Here's how the part is built. I have some questions about the finished solid (model axes, mm). A direction names the side the tool comes from. Coordinates: 2 decimals unless noted, no trailing zeros. Loops run counter-clockwise (first coordinate to the right, second up) from the corner with the lowest first, then second, coordinate; pieces in that order, holes last.
```python
from build123d import *

# Parameters (mm, degrees)
F0_R          = 15
F0_R_2        = 4
F1_DEPTH      = 2
F2_R          = 10.75
F2_R_2        = 4
F3_DEPTH      = 3
F4_R          = 1.5
F5_DEPTH      = 25
F5_DEPTH_BACK = 25
F6_R          = 1
F7_DEPTH      = 25


with BuildPart() as f1:
    # F0 (on Top) → F1 (new body)
    with BuildSketch(Plane.XY):
        Circle(F0_R)
        Circle(F0_R_2, mode=Mode.SUBTRACT)
    extrude(amount=F1_DEPTH)

    # F2 (on face) → F3 (join)
    with BuildSketch(Plane.XY.offset(2)):
        Circle(F2_R)
        Circle(F2_R_2, mode=Mode.SUBTRACT)
    extrude(amount=F3_DEPTH)

    # F4 (on Right) → F5 (cut, two sides)
    with BuildSketch(Plane.YZ) as f5_sk:
        with Locations((0, 2.5)):
            Circle(F4_R)
    extrude(amount=-F5_DEPTH, mode=Mode.SUBTRACT)
    extrude(f5_sk.sketch, amount=F5_DEPTH_BACK, mode=Mode.SUBTRACT)

    # F6 (on face) → F7 (cut)
    with BuildSketch(Plane.XY.offset(5)):
        with Locations((8.0107347155, -4.6250004669)):
            Circle(F6_R)
        with Locations((0, 9.25)):
            Circle(F6_R)
        with Locations((-8.0107355241, -4.6249990662)):
            Circle(F6_R)
    extrude(amount=-F7_DEPTH, mode=Mode.SUBTRACT)


solid = f1.part
```
1. I need wall thicknesses on line 1 along Y through (x, z) = (0, 2.5); line 2 along Y through (x, z) = (0, 1.6); line 3 along X through (y, z) = (-5.5, 1.2). Which ranges of each line are inside material? Lowest first, please.
2. I want a section at C-C (y = 0). Please give me the cut outline in (x, z), then the cut area to 3 significant figures.
3. We'd pull the mould along Z, two halves only. Please class faces 1 (the flat face through (3, -3, 0)), 2 (the cylindrical face through (8.02, 0.69, 1.17)), 3 (the flat face through (0, -5, 5)): +Z half, -Z half, draft (parallel to the pull), parting line (faces both ways), or undercut.
4. I want a section at D-D (y = 9.25). Please give me the cut outline in (x, z), then the cut area to 3 significant figures.
5. On a 3-axis mill with a long thin cutter (end or side, diameter ignored), from which of +Z, -Z, +X, -X, +Y, -Y can I reach the whole of each face in a straight line? I mean faces 4 (the cylindrical face through (7.01, -4.58, 2.54)), 5 (the flat face through (0, 11, 2)), 6 (the cylindrical face through (10.254, 3.229, 3.479)), 7 (the flat face through (0, -11, 2)). Say none if no direction works.
6. I want a section at B-B (z = 1.65). Please give me the cut outline in (x, y) (3 decimals).
7. I want a section at A-A (x = 0). Please give me the cut outline in (y, z), then the cut area to 3 significant figures.
Response values:
1. line 1: y = -10.75 to -4, 4 to 8.25, 10.25 to 10.75
1. line 2: y = -15 to -4, 4 to 8.25, 10.25 to 15
1. line 3: x = -13.96 to -8.49, -7.53 to 7.53, 8.49 to 13.96
2. outline: (-15, 0) - (-4, 0) - (-4, 1) - (-15, 1) - close; (-10.75, 4) - (-4, 4) - (-4, 5) - (-10.75, 5) - close; (4, 0) - (15, 0) - (15, 1) - (4, 1) - close; (4, 4) - (10.75, 4) - (10.75, 5) - (4, 5) - close
2. area: 35.5 mm2
3. face 1: -Z half
3. face 2: undercut
3. face 3: +Z half
4. outline: (-11.81, 0) - (-1, 0) - (-1, 5) - (-5.48, 5) - (-5.48, 2) - (-11.81, 2) - close; (1, 0) - (11.81, 0) - (11.81, 2) - (5.48, 2) - (5.48, 5) - (1, 5) - close
4. area: 70.1 mm2
5. face 4: +Z, -Z
5. face 5: +Z, +Y
5. face 6: +Z
5. face 7: +Z, -Y
6. outline: (-14.949, -1.236) arc R15 ccw to (14.949, -1.236) - (3.804, -1.236) arc R4 cw to (-3.804, -1.236) - close; (-14.949, 1.236) - (-3.804, 1.236) arc R4 cw to (3.804, 1.236) - (14.949, 1.236) arc R15 ccw to start; hole circle Ø2 at (-8.011, -4.625); hole circle Ø2 at (0, 9.25); hole circle Ø2 at (8.011, -4.625)
7. outline: (-15, 0) - (-4, 0) - (-4, 5) - (-10.75, 5) - (-10.75, 2) - (-15, 2) - close; (4, 0) - (8.25, 0) - (8.25, 5) - (4, 5) - close; (10.25, 0) - (15, 0) - (15, 2) - (10.75, 2) - (10.75, 5) - (10.25, 5) - close
7. area: 74.5 mm2
